Could you check a few things on this model? Use its own coordinates, in mm. Round coordinates to 2 decimals unless told otherwise and drop trailing zeros. Loops run counter-clockwise (first coordinate to the right, second up) from the corner with the lowest first, then second, coordinate; pieces in that order, holes last. Notation, with made-up numbers: (74.25, 88.25) -> (81.25, 88.25) arc R14 cw to (81.25, 95.25) -> close; hole circle Ø1 at (56, 50.5). An arc over 180 degrees is marked (long way). Write each question's results on one line, items separated by ' | '.
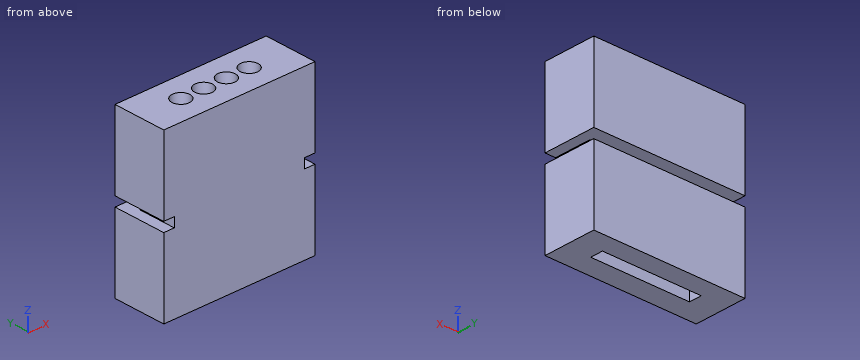
from build123d import *

# Parameters (mm, degrees)
BOSS_EXTRUDE1_DEPTH   = 5
SKETCH2_W             = 12.4
SKETCH2_H             = 0.9
CUT_EXTRUDE1_DEPTH    = 1.5
CROQUIS1_R            = 0.85
CORTAR_EXTRUIR1_DEPTH = 3
CROQUIS2_W            = 9.4
CROQUIS2_H            = 1.2
CORTAR_EXTRUIR2_DEPTH = 7.5


with BuildPart() as part:
    # Sketch1 → Boss-Extrude1 (new body)
    with BuildSketch(Plane(origin=(0, 0, 0), x_dir=(1, 0, 0), z_dir=(0, 1, 0))):
        Polygon((-7.2, -7.75), (7.2, -7.75), (7.2, -0.45), (6.2, -0.45), (6.2, 0.45), (7.2, 0.45), (7.2, 7.75), (-7.2, 7.75), (-7.2, 0.45), (-6.2, 0.45), (-6.2, -0.45), (-7.2, -0.45), align=None)
    extrude(amount=BOSS_EXTRUDE1_DEPTH)

    # Sketch2 → Cut-Extrude1 (cut)
    with BuildSketch(Plane(origin=(0, 5, 0), x_dir=(1, 0, 0), z_dir=(0, 1, 0))):
        Rectangle(SKETCH2_W, SKETCH2_H)
    extrude(amount=-CUT_EXTRUDE1_DEPTH, mode=Mode.SUBTRACT)

    # Croquis1 → Cortar-Extruir1 (cut)
    with BuildSketch(Plane.XY.offset(7.75)):
        with Locations((-3.25, 2.5)):
            Circle(CROQUIS1_R)
        with Locations((-1.083333333, 2.5)):
            Circle(CROQUIS1_R)
        with Locations((1.083333333, 2.5)):
            Circle(CROQUIS1_R)
        with Locations((3.25, 2.5)):
            Circle(CROQUIS1_R)
    extrude(amount=-CORTAR_EXTRUIR1_DEPTH, mode=Mode.SUBTRACT)

    # Croquis2 → Cortar-Extruir2 (cut)
    with BuildSketch(Plane(origin=(0, 0, -7.75), x_dir=(-1, 0, 0), z_dir=(0, 0, -1))):
        with Locations((0, 2.6)):
            Rectangle(CROQUIS2_W, CROQUIS2_H)
    extrude(amount=-CORTAR_EXTRUIR2_DEPTH, mode=Mode.SUBTRACT)


solid = part.part
1) I want a section at D-D, the plane z = -2. Write out the boundary of the cut face in (x, y), plus the area to 3 significant figures.
Model answer:
outline: (-7.2, 0) -> (7.2, 0) -> (7.2, 5) -> (-7.2, 5) -> close; hole (-4.7, 2) -> (4.7, 2) -> (4.7, 3.2) -> (-4.7, 3.2) -> close | area: 60.7 mm2
2) I need wall thicknesses on line 1 (X direction, y = 3, z = -2.25); line 2 (Z direction, x = 0.25, y = 3.55); line 3 (X direction, y = 1.85, z = 5.25). Which ranges of each line are inside material? Lowest first, please.
Model answer:
line 1: x = -7.2 to -4.7, 4.7 to 7.2 | line 2: z = -7.75 to -0.45, 0.45 to 7.75 | line 3: x = -7.2 to -3.8, -2.7 to -1.63, -0.54 to 0.54, 1.63 to 2.7, 3.8 to 7.2
3) I'm going to push flat-ended pins straight in: pin 1 (0.7 mm diameter, centred on y = 1, z = 0, fed in from -X); pin 2 (0.8 mm diameter, centred on x = -1.5, y = 2.5, fed in from +Z). Where does each tip first touch, or does it pass through?
Model answer:
pin 1: stops at x = -6.2 | pin 2: stops at z = 4.75
4) I want a section at A-A, the plane y = 4.55. Write out the boundary of the cut face in (x, z), plus the area to 3 significant figures.
Model answer:
outline: (-7.2, -7.75) -> (7.2, -7.75) -> (7.2, -0.45) -> (-7.2, -0.45) -> close; (-7.2, 0.45) -> (7.2, 0.45) -> (7.2, 7.75) -> (-7.2, 7.75) -> close | area: 210 mm2
5) I want a section at B-B, the plane z = 5.5. Write out the boundary of the cut face in (x, y).
Model answer:
outline: (-7.2, 0) -> (7.2, 0) -> (7.2, 5) -> (-7.2, 5) -> close; hole circle Ø1.7 at (-3.25, 2.5); hole circle Ø1.7 at (-1.08, 2.5); hole circle Ø1.7 at (1.08, 2.5); hole circle Ø1.7 at (3.25, 2.5)
6) I want a section at C-C, the plane x = 0. Write out the boundary of the cut face in (y, z).
Model answer:
outline: (0, -7.75) -> (2, -7.75) -> (2, -0.25) -> (3.2, -0.25) -> (3.2, -7.75) -> (5, -7.75) -> (5, -0.45) -> (3.5, -0.45) -> (3.5, 0.45) -> (5, 0.45) -> (5, 7.75) -> (0, 7.75) -> close
